Can you work these out from the model? Positions are in its coordinate system, mm. Face numbers are marked on the shaded views. A direction names the side the tool comes from. Coordinates: 2 decimals unless noted, no trailing zeros. Write each loop counter-clockwise with the first axis right and the second up, starting at its lowest first coordinate (ties: lowest second). Pieces come first, ordered by that corner, then holes. Notation, with made-up numbers: (26.5, -19) -> (44.5, -19) arc R14 ccw to (44.5, -13) -> close; hole circle Ø6 at (57, 71.5). An arc over 180 degrees is marked (long way). Use one line per item in the form item = value.
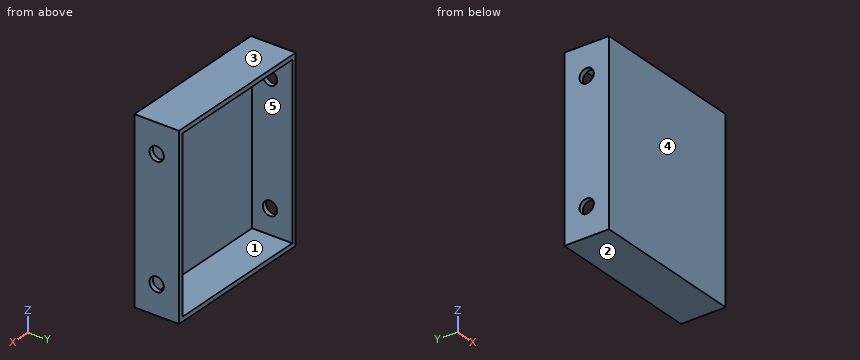
```python
from build123d import *

# Parameters (mm, degrees)
SKETCH_1_W          = 35
SKETCH_1_H          = 40
EXTRUDE_1_DEPTH     = 10
SHELL_1_T           = -1
SKETCH_2_R          = 1.6
CUT_EXTRUDE_1_DEPTH = 55.083269132


with BuildPart() as part:
    # 草图1 → 凸台-拉伸1 (new body)
    with BuildSketch(Plane(origin=(0, 0, 0), x_dir=(1, 0, 0), z_dir=(0, 1, 0))):
        with Locations((17.5, 20)):
            Rectangle(SKETCH_1_W, SKETCH_1_H)
    extrude(amount=EXTRUDE_1_DEPTH)

    # 抽壳1
    shell_1_openings = [part.faces().sort_by_distance(p)[0] for p in [
        (17.5, 10, -20),
    ]]
    offset(amount=SHELL_1_T, openings=shell_1_openings, kind=Kind.INTERSECTION)

    # 草图2 → 切除-拉伸1 (cut, through all)
    with BuildSketch(Plane.ZY):
        with Locations((-33.5, 5)):
            Circle(SKETCH_2_R)
        with Locations((-6.5, 5)):
            Circle(SKETCH_2_R)
    extrude(amount=-CUT_EXTRUDE_1_DEPTH, mode=Mode.SUBTRACT)


solid = part.part
```
Q1. Suppose I cut it at C-C (x = 23.5). Write out the boundary of the cut face in (y, z).
Return value:
outline = (0, -40) -> (10, -40) -> (10, -39) -> (1, -39) -> (1, -1) -> (10, -1) -> (10, 0) -> (0, 0) -> close
Q2. Suppose I cut it at B-B (z = -6.5). Write out the boundary of the cut face in (x, y).
Return value:
outline = (0, 0) -> (35, 0) -> (35, 3.4) -> (34, 3.4) -> (34, 1) -> (1, 1) -> (1, 3.4) -> (0, 3.4) -> close; (0, 6.6) -> (1, 6.6) -> (1, 10) -> (0, 10) -> close; (34, 6.6) -> (35, 6.6) -> (35, 10) -> (34, 10) -> close
Q3. Will these pins go through, and if not, where does the flat tip stop? pin 1 (4 mm diameter, centred on x = 13, z = -5, fed in from +Y); pin 2 (2.5 mm diameter, centred on y = 5, z = -33.5, fed in from +X).
Return value:
pin_1 = 1
pin_2 = through
Q4. Suppose I cut it at D-D (y = 5). Write out the boundary of the cut face in (x, z).
Return value:
outline = (0, -40) -> (35, -40) -> (35, -35.1) -> (34, -35.1) -> (34, -39) -> (1, -39) -> (1, -35.1) -> (0, -35.1) -> close; (0, -31.9) -> (1, -31.9) -> (1, -8.1) -> (0, -8.1) -> close; (0, -4.9) -> (1, -4.9) -> (1, -1) -> (34, -1) -> (34, -4.9) -> (35, -4.9) -> (35, 0) -> (0, 0) -> close; (34, -31.9) -> (35, -31.9) -> (35, -8.1) -> (34, -8.1) -> close
Q5. Thinking about a two-plate mould opening in Z: for the marked faces 3, 4 and 5, which applies, released by +Z, released by -Z, zero draft, split by the parting line, or undercut?
Return value:
face_3 = released by +Z
face_4 = zero draft
face_5 = undercut
Q6. For the marked faces 1 and 2, which set-ups out of +Z, -Z, +X, -X, +Y, -Y let a thin tool reach every point of the face, with its end or its side?
Return value:
face_1 = +Y
face_2 = -Z, +X, -X, +Y, -Y
Q7. Suppose I cut it at A-A (y = 8). Write out the boundary of the cut face in (x, z), then the cut area to 3 significant figures.
Return value:
outline = (0, -40) -> (35, -40) -> (35, 0) -> (0, 0) -> close; hole (1, -39) -> (34, -39) -> (34, -1) -> (1, -1) -> close
area = 146 mm2
Q8. If I drill on line 1 (X direction, y = 4.25, z = -30); line 2 (Z direction, x = 20, y = 9.5); line 3 (Y direction, x = 34.4, z = -6.5), over which ranges is the centre line in solid material (lowest first)? Write a range as from..to.
Return value:
line_1 = 0..1, 34..35
line_2 = -40..-39, -1..0
line_3 = 0..3.4, 6.6..10
